```python
from build123d import *

# Parameters (mm, degrees)
F0_W     = 27.6
F0_H     = 26.62
F1_DEPTH = 0.8
F2_W     = 27.6
F2_H     = 26.62
F2_W_2   = 26
F2_H_2   = 25.02
F3_DEPTH = 8
F4_R     = 0.95
F5_DEPTH = 5
F6_W     = 19.6
F6_H     = 4
F7_DEPTH = 1.7


with BuildPart() as f1:
    # F0 (on Front) → F1 (new body)
    with BuildSketch(Plane.XZ):
        Rectangle(F0_W, F0_H)
    extrude(amount=F1_DEPTH)

    # F2 (on face) → F3 (join)
    with BuildSketch(Plane.XZ.offset(0.8)):
        Rectangle(F2_W, F2_H)
        Rectangle(F2_W_2, F2_H_2, mode=Mode.SUBTRACT)
    extrude(amount=F3_DEPTH)

    # F4 (on face) → F5 (join)
    with BuildSketch(Plane.XZ.offset(0.8)):
        with Locations((-10.5, 9.99)):
            Circle(F4_R)
        with Locations((-10.5, -2.51)):
            Circle(F4_R)
        with Locations((10.5, 9.99)):
            Circle(F4_R)
        with Locations((10.5, -2.51)):
            Circle(F4_R)
    extrude(amount=F5_DEPTH)

    # F6 (on face) → F7 (cut)
    with BuildSketch(Plane(origin=(0, 0, -13.31), x_dir=(1, 0, 0), z_dir=(0, 0, -1))):
        with Locations((0, 4)):
            Rectangle(F6_W, F6_H)
    extrude(amount=-F7_DEPTH, mode=Mode.SUBTRACT)


solid = f1.part
```
Design review of the part built by this model. Coordinates are the model's own, in mm. A direction names the side the tool comes from. Give positions to 0.01 mm unless a question says otherwise; leave off trailing zeros. Order: outer loops, then holes, each group sorted by start corner. A loop starts at its lowest first (then second) coordinate and runs counter-clockwise, first axis right, second up. Notation, with made-up numbers: (6, 18.25) -> (49, 18.25) arc R12 ccw to (49, 31.25) -> close; hole circle Ø9 at (87, -24.5). An arc over 180 degrees is marked (long way). Write each question's results on one line, items separated by ' | '. Start each with the question number.
Q1. Machinability: for faces 1 (the flat face through (-11, -5.8, -2)), 2 (the flat face through (-1, -8.8, -13)), 3 (the flat face through (0, -6, -13)), which of the approach directions +Z, -Z, +X, -X, +Y, -Y give a long, thin tool a straight path to every point of the face, cutting with its end or side? Answer none if there is none.
Q2. For pin 1 (2 mm diameter, centred on x = 10.5, z = 10, fed in from -Y); pin 2 (1.5 mm diameter, centred on x = -5, z = -10.5, fed in from -Y), all flat-tipped, find the tip position at first contact; note any pin that passes through.
Q3. Wall thickness on L1, parallel to X at y = -1.5, z = -2.5; L2, parallel to Z at x = 12.75, y = -1; L3, parallel to X at y = -1, z = -11: over which ranges is each line inside the solid? List them lowest first. Write a range as from..to.
Q4. Add section D-D on z = -11. Give the boundary of the cut face in (x, y), and give its area (3 significant figures).
Q5. Add section A-A on x = 6.5. Give the boundary of the cut face in (y, z), and give its area (3 significant figures).
Q6. Mouldability with a two-part tool opening along Z and no side actions: class faces 4 (the flat face through (0, -4, 13.31)), 5 (the flat face through (10, -5.8, -2)), 6 (the flat face through (-13.8, -4, 0)) as +Z half, -Z half, draft (parallel to the pull), parting line (faces both ways), or undercut.
Q7. Add section C-C on y = -7.75. Give the boundary of the cut face in (x, z), and give its area (3 significant figures).
Q8. Add section B-B on x = -10.5. Give the boundary of the cut face in (y, z).
Found:
1) face 1: -Y | face 2: +Z, -Z, +X, -X, -Y | face 3: -Z
2) pin 1: stops at y = -5.8 | pin 2: stops at y = -0.8
3) L1: x = -13.8..-13, -11.45..-9.55, 9.55..11.45, 13..13.8 | L2: z = -13.31..-12.51, 12.51..13.31 | L3: x = -13.8..-13, 13..13.8
4) outline: (-13.8, -8.8) -> (-13, -8.8) -> (-13, -0.8) -> (13, -0.8) -> (13, -8.8) -> (13.8, -8.8) -> (13.8, 0) -> (-13.8, 0) -> close | area: 34.9 mm2
5) outline: (-8.8, -13.31) -> (-6, -13.31) -> (-6, -12.51) -> (-8.8, -12.51) -> close; (-8.8, 12.51) -> (-0.8, 12.51) -> (-0.8, -12.51) -> (-2, -12.51) -> (-2, -13.31) -> (0, -13.31) -> (0, 13.31) -> (-8.8, 13.31) -> close | area: 30.9 mm2
6) face 4: +Z half | face 5: undercut | face 6: draft
7) outline: (-13.8, -13.31) -> (13.8, -13.31) -> (13.8, 13.31) -> (-13.8, 13.31) -> close; hole (-13, -12.51) -> (13, -12.51) -> (13, 12.51) -> (-13, 12.51) -> close | area: 84.2 mm2
8) outline: (-8.8, -13.31) -> (0, -13.31) -> (0, 13.31) -> (-8.8, 13.31) -> (-8.8, 12.51) -> (-0.8, 12.51) -> (-0.8, 10.94) -> (-5.8, 10.94) -> (-5.8, 9.04) -> (-0.8, 9.04) -> (-0.8, -1.56) -> (-5.8, -1.56) -> (-5.8, -3.46) -> (-0.8, -3.46) -> (-0.8, -12.51) -> (-8.8, -12.51) -> close
